Geometry check sheet. Reference: the model listing, model coordinates, mm. Face numbers are marked on the shaded views. A direction names the side the tool comes from. Coordinates: 2 decimals unless noted, no trailing zeros. Write each loop counter-clockwise with the first axis right and the second up, starting at its lowest first coordinate (ties: lowest second). Pieces come first, ordered by that corner, then holes.
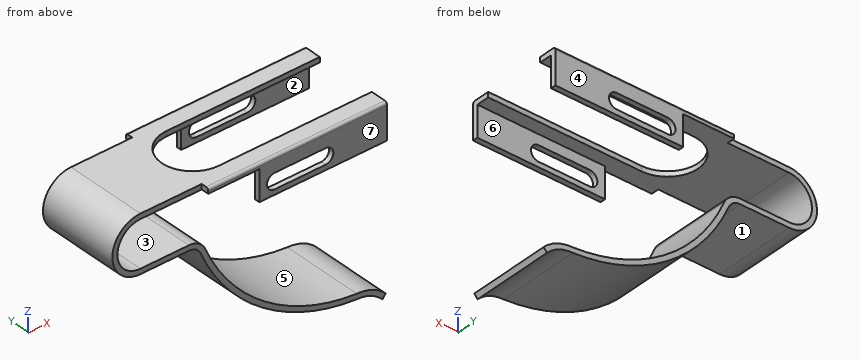
from build123d import *

# Parameters (mm, degrees)
F1_DEPTH  = 16
F2_W      = 70
F2_H      = 3
F3_DEPTH  = 2
F4_W      = 50
F4_H      = 14
F5_DEPTH  = 2
F6_R      = 1
F9_DEPTH  = 2
F11_DEPTH = 38.001


with BuildPart() as f1:
    # F0 (on Front) → F1 (new body)
    with BuildSketch(Plane.XZ):
        with BuildLine():
            Line((94, 11), (0, 11))
            ThreePointArc((0, 11), (-11, 0), (0, -11))
            Line((0, -11), (19, -11))
            ThreePointArc((19, -11), (21.768112, -11.836161), (23.61039, -14.064979))
            ThreePointArc((23.61039, -14.064979), (47.922303, -44.625558), (84.612543, -57.998828))
            ThreePointArc((84.612543, -57.998828), (90.151136, -59.22276), (94.749536, -62.543715))
            Line((94.749536, -62.543715), (96.044866, -61))
            ThreePointArc((96.044866, -61), (90.877978, -57.357164), (84.703426, -56))
            ThreePointArc((84.703426, -56), (49.067219, -42.985418), (25.454545, -13.29097))
            ThreePointArc((25.454545, -13.29097), (22.875357, -10.170626), (19, -9))
            Line((19, -9), (0, -9))
            ThreePointArc((0, -9), (-9, 0), (0, 9))
            Line((0, 9), (94, 9))
            Line((94, 9), (94, 11))
        make_face()
    extrude(amount=F1_DEPTH)

    # F2 (on face) → F3 (join)
    with BuildSketch(Plane.XY.offset(11)):
        with Locations((59, -17.5)):
            Rectangle(F2_W, F2_H)
    extrude(amount=-F3_DEPTH)

    # F4 (on face) → F5 (join)
    with BuildSketch(Plane.XZ.offset(19)):
        with Locations((69, 4)):
            Rectangle(F4_W, F4_H)
    extrude(amount=-F5_DEPTH)

    # F6
    f6_edges = [f1.edges().sort_by_distance(p)[0] for p in [
        (59, -19, 11),
    ]]
    fillet(f6_edges, radius=F6_R)

    # F7: F1 across plane


with BuildPart() as f1_1:
    add(f1.part)
    add(f1.part.mirror(Plane.XZ))

    # F8 (on face) → F9 (cut)
    with BuildSketch(Plane.XY.offset(11)):
        with BuildLine():
            Line((94, 12), (34, 12))
            ThreePointArc((34, 12), (22, 0), (34, -12))
            Line((34, -12), (94, -12))
            Line((94, -12), (94, 12))
        make_face()
    extrude(amount=-F9_DEPTH, mode=Mode.SUBTRACT)

    # F10 (on face) → F11 (cut, through all)
    with BuildSketch(Plane.XZ.offset(19)):
        with BuildLine():
            ThreePointArc((50, 5), (47, 2), (50, -1))
            Line((50, -1), (70, -1))
            ThreePointArc((70, -1), (73, 2), (70, 5))
            Line((70, 5), (50, 5))
        make_face()
    extrude(amount=-F11_DEPTH, mode=Mode.SUBTRACT)


solid = f1_1.part
1. Sectioned sample at A-A, the plane x = 13. Record the boundary of the cut face in (y, z), and give its area (3 significant figures).
Computed values:
outline: (-16, -11) - (16, -11) - (16, -9) - (-16, -9) - close; (-16, 9) - (16, 9) - (16, 11) - (-16, 11) - close
area: 128 mm2
2. Sectioned sample at C-C, the plane y = 0. Record the boundary of the cut face in (x, z).
Computed values:
outline: (0, -11) - (19, -11) arc R5 cw to (23.61, -14.06) arc R72 ccw to (84.61, -58) arc R14 cw to (94.75, -62.54) - (96.04, -61) arc R16 ccw to (84.7, -56) arc R70 cw to (25.45, -13.29) arc R7 ccw to (19, -9) - (0, -9) arc R9 cw to (0, 9) - (22, 9) - (22, 11) - (0, 11) arc R11 ccw to start
3. Sectioned sample at B-B, the plane x = 40.5. Record the boundary of the cut face in (y, z).
Computed values:
outline: (-19, 9) - (-12, 9) - (-12, 11) - (-18, 11) arc R1 ccw to (-19, 10) - close; (-16, -38.49) - (16, -38.49) - (16, -35.7) - (-16, -35.7) - close; (12, 9) - (19, 9) - (19, 10) arc R1 ccw to (18, 11) - (12, 11) - close
4. Thickness scan on line 1 along Z through (x, y) = (19, -15.5); line 2 along Y through (x, z) = (73, 4); line 3 along X through (y, z) = (-3, 0). Record the ranges inside material, lowest first.
Computed values:
line 1: z = -11 to -9, 9 to 11
line 2: y = -19 to -17, 17 to 19
line 3: x = -11 to -9
5. Draft check along Y on the marked faces 5, 6 and 7. Enter one of: released by +Y, released by -Y, zero draft, split by the parting line, or undercut.
Computed values:
face 5: zero draft
face 6: undercut
face 7: released by -Y
6. Access from +Z, -Z, +X, -X, +Y, -Y to the whole of each face (thin tool, end or side, straight path). Record for the marked faces 1, 2, 3 and 4.
Computed values:
face 1: -Z, -X, +Y, -Y
face 2: -Z, +X, -X
face 3: +X, +Y, -Y
face 4: +Z, -Z, +X, -X, +Y
7. Gauge pin test, flat ends, axial feed: pin 1 Ø15 at (x, y) = (8.5, 1.5) entering from -Z; pin 2 Ø12 at (y, z) = (-3, -49) entering from -X; pin 3 Ø1 at (x, y) = (45, -1) entering from -Z. Record the tip position at first contact, or that the pin passes through.
Computed values:
pin 1: stops at z = -11
pin 2: stops at x = 45.75
pin 3: stops at z = -42.8
8. Sectioned sample at D-D, the plane x = 66.5. Record the boundary of the cut face in (y, z), and give its area (3 significant figures).
Computed values:
outline: (-19, -3) - (-17, -3) - (-17, -1) - (-19, -1) - close; (-19, 5) - (-17, 5) - (-17, 9) - (-12, 9) - (-12, 11) - (-18, 11) arc R1 ccw to (-19, 10) - close; (-16, -54.26) - (16, -54.26) - (16, -52.14) - (-16, -52.14) - close; (12, 9) - (17, 9) - (17, 5) - (19, 5) - (19, 10) arc R1 ccw to (18, 11) - (12, 11) - close; (17, -3) - (19, -3) - (19, -1) - (17, -1) - close
area: 119 mm2
